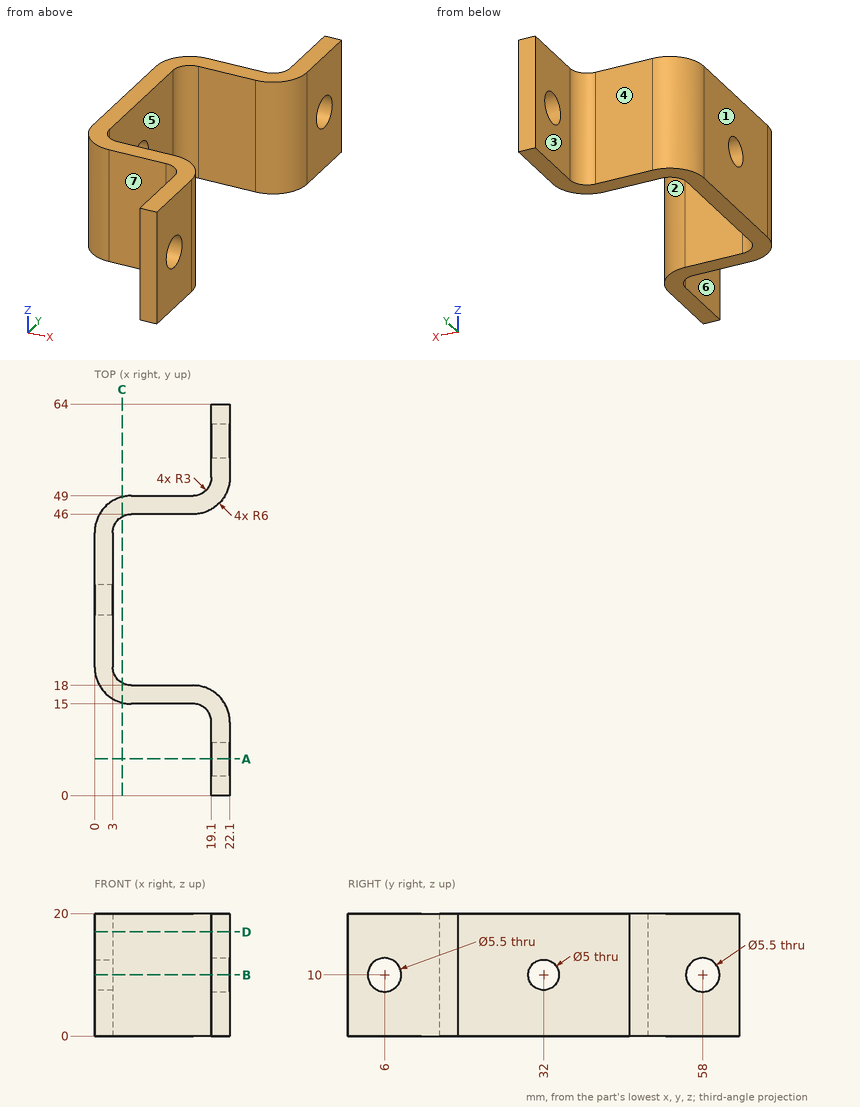
Check sheet for the drawn part. Datum: minimum x, y, z corner. Units: mm. A direction names the side the tool comes from. Give positions to 0.01 mm unless a question says otherwise; leave off trailing zeros. Write each loop counter-clockwise with the first axis right and the second up, starting at its lowest first coordinate (ties: lowest second). Pieces come first, ordered by that corner, then holes. Notation, with made-up numbers: M 24,49 L 60,49 A26 cw 60,88 Z; hole C 29.5,-32.5 d11. An arc over 180 degrees is marked long. One line per question, with ' | ' between items.
1. Cross-section at C-C (x = 4.5). Enter the section's corners in (y, z).
Ans:
outline: M 15.19,0 L 18.4,0 L 18.4,20 L 15.19,20 Z; M 45.6,0 L 48.81,0 L 48.81,20 L 45.6,20 Z
2. Cross-section at A-A (y = 6). Enter the section's corners in (x, z), plus the area to 3 significant figures.
Ans:
outline: M 19.1,0 L 22.1,0 L 22.1,7.25 L 19.1,7.25 Z; M 19.1,12.75 L 22.1,12.75 L 22.1,20 L 19.1,20 Z | area: 43.5 mm2
3. Scan lines: line 1 along Y through (x, z) = (9.5, 4); line 2 along Y through (x, z) = (19.9, 10); line 3 along X through (y, z) = (22, 14). Record each from-to range of solid material in increasing order. Write a range as from..to.
Ans:
line 1: 15..18, 46..49 | line 2: 0..3.25, 8.75..16.64, 47.36..55.25, 60.75..64 | line 3: 0..3
4. Cross-section at B-B (z = 10). Count the separate pieces of the cut face and the enclosed holes in it, plus the area to 3 significant figures.
Ans:
separate pieces: 4 | enclosed holes: 0 | area: 235 mm2
5. Cross-section at D-D (z = 17). Enter the section's corners in (x, y).
Ans:
outline: M 0,21 A6 ccw 6,15 L 16.1,15 A3 cw 19.1,12 L 19.1,0 L 22.1,0 L 22.1,12 A6 ccw 16.1,18 L 6,18 A3 cw 3,21 L 3,43 A3 cw 6,46 L 16.1,46 A6 ccw 22.1,52 L 22.1,64 L 19.1,64 L 19.1,52 A3 cw 16.1,49 L 6,49 A6 ccw 0,43 Z
6. Gauge pin test, flat ends, axial feed: pin 1 (3 mm diameter, centred on y = 38.5, z = 2.5, fed in from +X); pin 2 (11 mm diameter, centred on x = 13, z = 11.5, fed in from +Y); pin 3 (11 mm diameter, centred on x = 12, z = 12.5, fed in from +Y); pin 4 (4 mm diameter, centred on y = 32, z = 10, fed in from -X). Record the tip position at first contact, or that the pin passes through.
Ans:
pin 1: x = 3 | pin 2: y = 50.2 | pin 3: y = 49.35 | pin 4: through
7. Set-up check for the marked faces 1, 2 and 3: record each of +Z, -Z, +X, -X, +Y, -Y from which the full face is reachable in a straight line by a thin tool's end or side.
Ans:
face 1: +Z, -Z, -X, +Y, -Y | face 2: +Z, -Z, +X | face 3: +Z, -Z, -X, +Y
8. Mould release check, pull along Y, two halves, no side actions. Record for the marked faces 4, 5, 6 and 7: released by +Y, released by -Y, zero draft, split by the parting line, or undercut.
Ans:
face 4: released by +Y | face 5: undercut | face 6: zero draft | face 7: released by -Y
